Geometry check sheet. Reference: the model listing, model coordinates, mm. Face numbers are marked on the shaded views. A direction names the side the tool comes from. Coordinates: 2 decimals unless noted, no trailing zeros. Write each loop counter-clockwise with the first axis right and the second up, starting at its lowest first coordinate (ties: lowest second). Pieces come first, ordered by that corner, then holes. Notation, with made-up numbers: (10, 49.25) -> (20, 49.25) arc R34 cw to (20, 81.25) -> close; hole circle Ø7 at (61, 51.25). An arc over 180 degrees is marked (long way). Use a Markdown table: item, result.
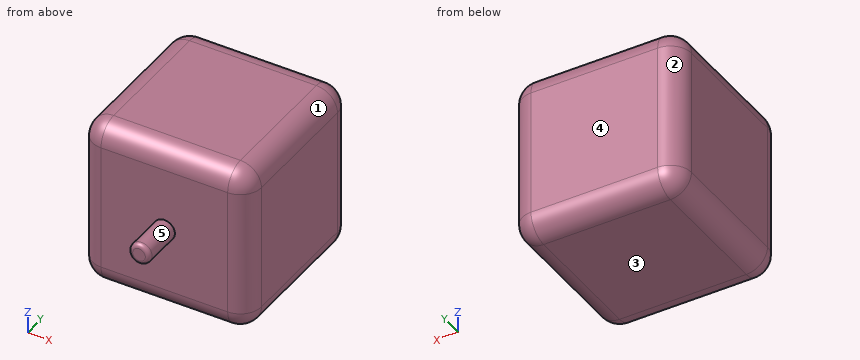
```python
from build123d import *

# Parameters (mm, degrees)
SKETCH1_W           = 80
SKETCH1_H           = 80
BOSS_EXTRUDE1_DEPTH = 80
SKETCH2_R           = 5
BOSS_EXTRUDE2_DEPTH = 20
FILLET1_R           = 10
FILLET2_R           = 2


with BuildPart() as part:
    # Sketch1 → Boss-Extrude1 (new body)
    with BuildSketch(Plane(origin=(0, 0, 0), x_dir=(1, 0, 0), z_dir=(0, 1, 0))):
        Rectangle(SKETCH1_W, SKETCH1_H)
    extrude(amount=BOSS_EXTRUDE1_DEPTH)

    # Sketch2 → Boss-Extrude2 (add)
    with BuildSketch(Plane.XZ):
        with Locations(Location((0, 0, 0), (0, 0, 90))):
            Circle(SKETCH2_R)
    extrude(amount=BOSS_EXTRUDE2_DEPTH)

    # Fillet1
    fillet1_edges = [part.edges().sort_by_distance(p)[0] for p in [
        (-40, 80, 0),
        (0, 80, 40),
        (40, 80, 0),
        (0, 0, 40),
        (-40, 0, 0),
        (0, 0, -40),
        (40, 0, 0),
        (40, 40, 40),
        (-40, 40, 40),
        (-40, 40, -40),
        (40, 40, -40),
        (0, 80, -40),
    ]]
    fillet(fillet1_edges, radius=FILLET1_R)

    # Fillet2
    fillet2_edges = [part.edges().sort_by_distance(p)[0] for p in [
        (0, -20, -5),
    ]]
    fillet(fillet2_edges, radius=FILLET2_R)


solid = part.part
```
Item 1: Mould release check, pull along Z, two halves, no side actions. Record for the marked faces 1, 2 and 3: +Z half, -Z half, draft (parallel to the pull), parting line (faces both ways), or undercut.
Answer block:
| item | result |
|---|---|
| face 1 | +Z half |
| face 2 | draft |
| face 3 | -Z half |
Item 2: Section check D-D on x = 0. Record the boundary of the cut face in (y, z), then the cut area to 3 significant figures.
Answer block:
| item | result |
|---|---|
| outline | (-20, -3) arc R2 ccw to (-18, -5) -> (0, -5) -> (0, -30) arc R10 ccw to (10, -40) -> (70, -40) arc R10 ccw to (80, -30) -> (80, 30) arc R10 ccw to (70, 40) -> (10, 40) arc R10 ccw to (0, 30) -> (0, 5) -> (-18, 5) arc R2 ccw to (-20, 3) -> close |
| area | 6,510 mm^2 |
Item 3: Section check A-A on x = 9.5. Record the boundary of the cut face in (y, z).
Answer block:
| item | result |
|---|---|
| outline | (0, -30) arc R10 ccw to (10, -40) -> (70, -40) arc R10 ccw to (80, -30) -> (80, 30) arc R10 ccw to (70, 40) -> (10, 40) arc R10 ccw to (0, 30) -> close |
Item 4: Section check C-C on z = 0. Record the boundary of the cut face in (x, y), then the cut area to 3 significant figures.
Answer block:
| item | result |
|---|---|
| outline | (-40, 10) arc R10 ccw to (-30, 0) -> (-5, 0) -> (-5, -18) arc R2 ccw to (-3, -20) -> (3, -20) arc R2 ccw to (5, -18) -> (5, 0) -> (30, 0) arc R10 ccw to (40, 10) -> (40, 70) arc R10 ccw to (30, 80) -> (-30, 80) arc R10 ccw to (-40, 70) -> close |
| area | 6,510 mm^2 |
Item 5: Section check B-B on y = 2. Record the boundary of the cut face in (x, z), then the cut area to 3 significant figures.
Answer block:
| item | result |
|---|---|
| outline | (-36, -30) arc R6 ccw to (-30, -36) -> (30, -36) arc R6 ccw to (36, -30) -> (36, 30) arc R6 ccw to (30, 36) -> (-30, 36) arc R6 ccw to (-36, 30) -> close |
| area | 5,150 mm^2 |
Item 6: Thickness scan on L1, parallel to Y at x = -8.5, z = 12.5; L2, parallel to Z at x = -4, y = -12; L3, parallel to Z at x = -35, y = 74. Record the ranges inside material, lowest first. Write a range as [from, to].
Answer block:
| item | result |
|---|---|
| L1 | y = [0, 80] |
| L2 | z = [-3, 3] |
| L3 | z = [-37.68, 37.68] |
Item 7: Tool access check on the marked faces 4 and 5. Record the directions out of +Z, -Z, +X, -X, +Y, -Y that give a thin tool (end or side, any length) a straight path to the whole face; none if there is none.
Answer block:
| item | result |
|---|---|
| face 4 | +Z, -Z, +X, -X, +Y |
| face 5 | -Y |
Item 8: Depth check by flat-ended pin: P1, Ø18, axis at x = 2.5, z = 6, coming from the -Y side; P2, Ø4, axis at x = 2, z = 28, coming from the -Y side. Enter the tip coordinate at first touch or a pass-through.
Answer block:
| item | result |
|---|---|
| P1 | stops at y = -20 |
| P2 | stops at y = 0 |
